from build123d import *

# Parameters (mm, degrees)
F0_R     = 6.35
F1_DEPTH = 12.7
F2_DEPTH = 203.2
F3_R     = 95
F3_R_2   = 4.5
F3_R_3   = 2.75
F3_R_4   = 30
F4_DEPTH = 6.35


with BuildPart() as f1:
    # F0 (on Top) → F1 (new body)
    with BuildSketch(Plane.XY):
        with BuildLine():
            Line((-127, -152.4), (127, -152.4))
            ThreePointArc((127, -152.4), (144.9605122421, -144.9605122421), (152.4, -127))
            Line((152.4, -127), (152.4, 127))
            ThreePointArc((152.4, 127), (144.9605122421, 144.9605122421), (127, 152.4))
            Line((127, 152.4), (-127, 152.4))
            ThreePointArc((-127, 152.4), (-144.9605122421, 144.9605122421), (-152.4, 127))
            Line((-152.4, 127), (-152.4, -127))
            ThreePointArc((-152.4, -127), (-144.9605122421, -144.9605122421), (-127, -152.4))
        make_face()
        with Locations((-127, -127)):
            Circle(F0_R, mode=Mode.SUBTRACT)
        with Locations((-63.5, -127)):
            Circle(F0_R, mode=Mode.SUBTRACT)
        with Locations((-127, -63.5)):
            Circle(F0_R, mode=Mode.SUBTRACT)
        with Locations((0, -127)):
            Circle(F0_R, mode=Mode.SUBTRACT)
        with Locations((63.5, -127)):
            Circle(F0_R, mode=Mode.SUBTRACT)
        with Locations((127, -127)):
            Circle(F0_R, mode=Mode.SUBTRACT)
        with Locations((127, -63.5)):
            Circle(F0_R, mode=Mode.SUBTRACT)
        with Locations((-127, 0)):
            Circle(F0_R, mode=Mode.SUBTRACT)
        with Locations((-127, 63.5)):
            Circle(F0_R, mode=Mode.SUBTRACT)
        with Locations((-127, 127)):
            Circle(F0_R, mode=Mode.SUBTRACT)
        with Locations((-63.5, 127)):
            Circle(F0_R, mode=Mode.SUBTRACT)
        with BuildLine():
            Line((107.95, 95.25), (107.95, -107.95))
            Line((107.95, -107.95), (101.6, -107.95))
            Line((101.6, -107.95), (-101.6, -107.95))
            Line((-101.6, -107.95), (-107.95, -107.95))
            Line((-107.95, -107.95), (-107.95, 95.25))
            ThreePointArc((-107.95, 95.25), (-104.2302561211, 104.2302561211), (-95.25, 107.95))
            Line((-95.25, 107.95), (95.25, 107.95))
            ThreePointArc((95.25, 107.95), (104.2302561211, 104.2302561211), (107.95, 95.25))
        make_face(mode=Mode.SUBTRACT)
        with Locations((125.8721500635, 0)):
            Circle(F0_R, mode=Mode.SUBTRACT)
        with Locations((127, 63.5)):
            Circle(F0_R, mode=Mode.SUBTRACT)
        with Locations((0, 127)):
            Circle(F0_R, mode=Mode.SUBTRACT)
        with Locations((63.5, 127)):
            Circle(F0_R, mode=Mode.SUBTRACT)
        with Locations((127, 127)):
            Circle(F0_R, mode=Mode.SUBTRACT)
        with BuildLine():
            Line((-101.6, -107.95), (101.6, -107.95))
            Line((101.6, -107.95), (101.6, 88.9))
            ThreePointArc((101.6, 88.9), (97.8802561211, 97.8802561211), (88.9, 101.6))
            Line((88.9, 101.6), (-88.9, 101.6))
            ThreePointArc((-88.9, 101.6), (-97.8802561211, 97.8802561211), (-101.6, 88.9))
            Line((-101.6, 88.9), (-101.6, -107.95))
        make_face()
        with Locations((-54.9926131403, -31.75)):
            Circle(F0_R, mode=Mode.SUBTRACT)
        with Locations((0, -63.5)):
            Circle(F0_R, mode=Mode.SUBTRACT)
        with Locations((54.9926131403, -31.75)):
            Circle(F0_R, mode=Mode.SUBTRACT)
        with Locations((-54.9926131403, 31.75)):
            Circle(F0_R, mode=Mode.SUBTRACT)
        with Locations((54.9926131403, 31.75)):
            Circle(F0_R, mode=Mode.SUBTRACT)
        with Locations((0, 63.5)):
            Circle(F0_R, mode=Mode.SUBTRACT)
    extrude(amount=F1_DEPTH)

    # F0 (on Top) → F2 (join)
    with BuildSketch(Plane.XY):
        with BuildLine():
            Line((101.6, -107.95), (107.95, -107.95))
            Line((107.95, -107.95), (107.95, 95.25))
            ThreePointArc((107.95, 95.25), (104.2302561211, 104.2302561211), (95.25, 107.95))
            Line((95.25, 107.95), (-95.25, 107.95))
            ThreePointArc((-95.25, 107.95), (-104.2302561211, 104.2302561211), (-107.95, 95.25))
            Line((-107.95, 95.25), (-107.95, -107.95))
            Line((-107.95, -107.95), (-101.6, -107.95))
            Line((-101.6, -107.95), (-101.6, 88.9))
            ThreePointArc((-101.6, 88.9), (-97.8802561211, 97.8802561211), (-88.9, 101.6))
            Line((-88.9, 101.6), (88.9, 101.6))
            ThreePointArc((88.9, 101.6), (97.8802561211, 97.8802561211), (101.6, 88.9))
            Line((101.6, 88.9), (101.6, -107.95))
        make_face()
    extrude(amount=F2_DEPTH)

    # F3 (on face) → F4 (join)
    with BuildSketch(Plane.XY.offset(203.2)):
        with BuildLine():
            Line((101.6, -107.95), (107.95, -107.95))
            Line((107.95, -107.95), (107.95, 95.25))
            ThreePointArc((107.95, 95.25), (104.2302561211, 104.2302561211), (95.25, 107.95))
            Line((95.25, 107.95), (-95.25, 107.95))
            ThreePointArc((-95.25, 107.95), (-104.2302561211, 104.2302561211), (-107.95, 95.25))
            Line((-107.95, 95.25), (-107.95, -107.95))
            Line((-107.95, -107.95), (-101.6, -107.95))
            Line((-101.6, -107.95), (-101.6, 88.9))
            ThreePointArc((-101.6, 88.9), (-97.8802561211, 97.8802561211), (-88.9, 101.6))
            Line((-88.9, 101.6), (88.9, 101.6))
            ThreePointArc((88.9, 101.6), (97.8802561211, 97.8802561211), (101.6, 88.9))
            Line((101.6, 88.9), (101.6, -107.95))
        make_face()
        with BuildLine():
            Line((-101.6, -107.95), (101.6, -107.95))
            Line((101.6, -107.95), (101.6, 88.9))
            ThreePointArc((101.6, 88.9), (97.8802561211, 97.8802561211), (88.9, 101.6))
            Line((88.9, 101.6), (-88.9, 101.6))
            ThreePointArc((-88.9, 101.6), (-97.8802561211, 97.8802561211), (-101.6, 88.9))
            Line((-101.6, 88.9), (-101.6, -107.95))
        make_face()
        Circle(F3_R, mode=Mode.SUBTRACT)
        Circle(F3_R)
        with Locations((-60.811183182, -60.811183182)):
            Circle(F3_R_2, mode=Mode.SUBTRACT)
        with Locations((0, -86)):
            Circle(F3_R_2, mode=Mode.SUBTRACT)
        with Locations((-32.9107751834, -79.453639796)):
            Circle(F3_R_2, mode=Mode.SUBTRACT)
        with Locations((-79.453639796, -32.9107751834)):
            Circle(F3_R_2, mode=Mode.SUBTRACT)
        with Locations((-34.8, -34.8)):
            Circle(F3_R_3, mode=Mode.SUBTRACT)
        with Locations((32.9107751834, -79.453639796)):
            Circle(F3_R_2, mode=Mode.SUBTRACT)
        with Locations((60.811183182, -60.811183182)):
            Circle(F3_R_2, mode=Mode.SUBTRACT)
        with Locations((34.8, -34.8)):
            Circle(F3_R_3, mode=Mode.SUBTRACT)
        with Locations((79.453639796, -32.9107751834)):
            Circle(F3_R_2, mode=Mode.SUBTRACT)
        with Locations((-86, 0)):
            Circle(F3_R_2, mode=Mode.SUBTRACT)
        with Locations((-79.453639796, 32.9107751834)):
            Circle(F3_R_2, mode=Mode.SUBTRACT)
        Circle(F3_R_4, mode=Mode.SUBTRACT)
        with Locations((-34.8, 34.8)):
            Circle(F3_R_3, mode=Mode.SUBTRACT)
        with Locations((-60.811183182, 60.811183182)):
            Circle(F3_R_2, mode=Mode.SUBTRACT)
        with Locations((-32.9107751834, 79.453639796)):
            Circle(F3_R_2, mode=Mode.SUBTRACT)
        with Locations((0, 86)):
            Circle(F3_R_2, mode=Mode.SUBTRACT)
        with Locations((34.8, 34.8)):
            Circle(F3_R_3, mode=Mode.SUBTRACT)
        with Locations((86, 0)):
            Circle(F3_R_2, mode=Mode.SUBTRACT)
        with Locations((79.453639796, 32.9107751834)):
            Circle(F3_R_2, mode=Mode.SUBTRACT)
        with Locations((32.9107751834, 79.453639796)):
            Circle(F3_R_2, mode=Mode.SUBTRACT)
        with Locations((60.811183182, 60.811183182)):
            Circle(F3_R_2, mode=Mode.SUBTRACT)
    extrude(amount=F4_DEPTH)


solid = f1.part
Geometry: final body of the model. Coordinates: model frame, mm. A direction names the side the tool comes from. Round coordinates to 2 decimals unless told otherwise and drop trailing zeros. Order: outer loops, then holes, each group sorted by start corner. A loop starts at its lowest first (then second) coordinate and runs counter-clockwise, first axis right, second up.
Q1. Section A-A, the plane z = 189.5. Output: boundary loops of the cut face in (x, y).
Result sheet:
outline: (-107.95, -107.95) - (-101.6, -107.95) - (-101.6, 88.9) arc R12.7 cw to (-88.9, 101.6) - (88.9, 101.6) arc R12.7 cw to (101.6, 88.9) - (101.6, -107.95) - (107.95, -107.95) - (107.95, 95.25) arc R12.7 ccw to (95.25, 107.95) - (-95.25, 107.95) arc R12.7 ccw to (-107.95, 95.25) - close
Q2. Access query for faces 1 (the face through (-0.59, 90.46, 206.33)), 2 (the face through (-101.6, -11, 107)), 3 (the face through (107.95, -8, 110)). Directions: +Z, -Z, +X, -X, +Y, -Y. A direction counts if a zero-diameter tool reaches every point of the face in a straight line with its end or side. Return the directions, or none.
Result sheet:
face 1: +Z
face 2: -Y
face 3: +Z, +X, +Y, -Y
Q3. Material intervals for probe 1 along Y at (x, z) = (0, 10); probe 2 along Z at (x, y) = (29.5, -50.5); probe 3 along X at (y, z) = (40.5, 45), sorted ascending.
Result sheet:
probe 1: y = -152.4 to -133.35, -120.65 to -69.85, -57.15 to 57.15, 69.85 to 120.65, 133.35 to 152.4
probe 2: z = 0 to 12.7, 203.2 to 209.55
probe 3: x = -107.95 to -101.6, 101.6 to 107.95
Q4. Mould query, pull axis Y, two halves, no side actions, for faces 4 (the face through (-144.76, 145.16, 6.26)), 5 (the face through (97.78, 97.98, 106.62)), 6 (the face through (-2, 2, 0)), 7 (the face through (-48.936, 33.657, 6.261)). Classes: released by +Y, released by -Y, zero draft, split by the parting line, or undercut.
Result sheet:
face 4: released by +Y
face 5: released by -Y
face 6: zero draft
face 7: undercut
Q5. Pin query (flat end, axial travel): pin 1 (2 mm diameter, centred on x = -13, z = 117, fed in from +Y); pin 2 (10 mm diameter, centred on x = 127, y = -63.5, fed in from -Z); pin 3 (1 mm diameter, centred on x = 45.5, z = 41.5, fed in from -Y); pin 4 (8 mm diameter, centred on x = 23, y = 0, fed in from +Z). Return the tip coordinate at first contact, or that it passes through.
Result sheet:
pin 1: stops at y = 107.95
pin 2: passes through
pin 3: stops at y = 101.6
pin 4: stops at z = 12.7
Q6. Section B-B, the plane x = -42. Output: boundary loops of the cut face in (y, z).
Result sheet:
outline: (-152.4, 0) - (152.4, 0) - (152.4, 12.7) - (107.95, 12.7) - (107.95, 209.55) - (-107.95, 209.55) - (-107.95, 203.2) - (101.6, 203.2) - (101.6, 12.7) - (-152.4, 12.7) - close
